from build123d import *

# Parameters (mm, degrees)
F1_DEPTH         = 50
F3_DEPTH         = 46
F5_DEPTH         = 25
F7_DEPTH         = 25
F8_W             = 3.4296980606
F8_H             = 1.9268138267
F9_DEPTH         = 25
F12_D            = 4
F12_DEPTH        = 16
F12_TIP          = 1.2017212381
F12_ON_F11_D     = 4
F12_ON_F11_DEPTH = 16
F12_ON_F11_TIP   = 1.2017212381
F13_R            = 5
F14_R            = 2
F15_R            = 5


with BuildPart() as f1:
    # F0 (on Right) → F1 (new body)
    with BuildSketch(Plane.YZ):
        Polygon((-50, 4), (-50, 0), (0, 0), (0, 50), (-4, 50), (-4, 4), align=None)
    extrude(amount=F1_DEPTH)

    # F2 (on face) → F3 (join)
    with BuildSketch(Plane.XZ.offset(4)):
        Polygon((25, 50), (24, 50), (24, 4), (26, 4), (26, 50), align=None)
    extrude(amount=F3_DEPTH)

    # F4 (on face) → F5 (cut)
    with BuildSketch(Plane(origin=(24, 0, 0), x_dir=(0, -1, 0), z_dir=(-1, 0, 0))):
        with BuildLine():
            Line((50, 50), (4, 50))
            add(Edge.make_bspline(
                [(4, 50), (18.2273147409, 34.0409380861), (26.0339638541, 8.7697255613), (37.7275896233, 4)],
                knots=[0, 0, 0, 0, 0.6888068808, 0.6888068808, 0.6888068808, 0.6888068808], degree=3))
            Line((37.7275896233, 4), (49.3700235132, 4))
            Line((49.3700235132, 4), (50, 4))
            Line((50, 4), (50, 50))
        make_face()
    extrude(amount=-F5_DEPTH, mode=Mode.SUBTRACT)

    # F6 (on face) → F7 (cut)
    with BuildSketch(Plane(origin=(24, 0, 0), x_dir=(0, -1, 0), z_dir=(-1, 0, 0))):
        with BuildLine():
            Line((4, 4), (20.8637948117, 4))
            add(Edge.make_bspline(
                [(20.8637948117, 4), (16.6060887277, 7.1307057515), (16.0147414533, 11.764077872), (13.590214774, 15.4687128961)],
                knots=[0, 0, 0, 0, 13.5807342238, 13.5807342238, 13.5807342238, 13.5807342238], degree=3))
            add(Edge.make_bspline(
                [(13.590214774, 15.4687128961), (8.6228903383, 18.1297790259), (5.6070159189, 17.9523732513), (4, 15.4687128961)],
                knots=[0, 0, 0, 0, 9.590214774, 9.590214774, 9.590214774, 9.590214774], degree=3))
            Line((4, 15.4687128961), (4, 4))
        make_face()
        Polygon((4, 33.209156245), (4, 24.3389345706), (10.5743389577, 24.3389345706), align=None)
    extrude(amount=-F7_DEPTH, mode=Mode.SUBTRACT)

    # F8 (on face) → F9 (cut)
    with BuildSketch(Plane(origin=(24, 0, 0), x_dir=(0, -1, 0), z_dir=(-1, 0, 0))):
        with Locations((5.7148490303, 16.4321198095)):
            Rectangle(F8_W, F8_H)
    extrude(amount=-F9_DEPTH, mode=Mode.SUBTRACT)

    # F12
    with Locations(Plane.XZ.offset(4)):
        with Locations((12.5, 27), (38, 27)):
            Hole(F12_D / 2, depth=F12_DEPTH)
            with Locations((0, 0, -(F12_DEPTH + F12_TIP / 2))):  # 118° drill point
                Cone(0, F12_D / 2, F12_TIP, mode=Mode.SUBTRACT)

    # F12 on F11
    with Locations(Plane.XY.offset(4)):
        with Locations((38, -27), (12, -27)):
            Hole(F12_ON_F11_D / 2, depth=F12_ON_F11_DEPTH)
            with Locations((0, 0, -(F12_ON_F11_DEPTH + F12_ON_F11_TIP / 2))):  # 118° drill point
                Cone(0, F12_ON_F11_D / 2, F12_ON_F11_TIP, mode=Mode.SUBTRACT)

    # F13
    f13_edges = [f1.edges().sort_by_distance(p)[0] for p in [
        (25, 0, 0),
    ]]
    fillet(f13_edges, radius=F13_R)

    # F14
    f14_edges = [f1.edges().sort_by_distance(p)[0] for p in [
        (25, -4, 4),
    ]]
    fillet(f14_edges, radius=F14_R)

    # F15
    f15_edges = [f1.edges().sort_by_distance(p)[0] for p in [
        (0, -2, 50),
        (50, -2, 50),
        (0, -50, 2),
        (50, -50, 2),
    ]]
    fillet(f15_edges, radius=F15_R)


solid = f1.part
Geometry check sheet. Reference: the model listing, model coordinates, mm. A direction names the side the tool comes from. Coordinates: 2 decimals unless noted, no trailing zeros. Order: outer loops, then holes, each group sorted by start corner. A loop starts at its lowest first (then second) coordinate and runs counter-clockwise, first axis right, second up. Notation, with made-up numbers: (-18, 43) - (27, 43) arc R11 cw to (27, 56) - close; hole circle Ø4 at (11.5, 63). An arc over 180 degrees is marked (long way). Answer in a Markdown table with one row per item. Add a question column.
1) Cross-section at C-C, the plane y = -27. State how many separate pieces and enclosed holes the cut face has, then the cut area to 3 significant figures.
2) Material ranges on line 1 along Y through (x, z) = (10.5, 38.5); line 2 along Z through (x, y) = (15, -7.5); line 3 along Z through (x, y) = (12, -1), recorded low to high. Write a range as [from, to].
3) Set-up check for faces 4 (the flat face through (25, -6, 17.396)), 5 (the cylindrical face through (1, -48, 2)), 6 (the flat face through (24, -16, 24)): record each of +Z, -Z, +X, -X, +Y, -Y from which the full face is reachable in a straight line by a thin tool's end or side.
4) Cross-section at B-B, the plane x = 15.5. Record the cut outline in (y, z), then the cut area to 3 significant figures.
5) Cross-section at A-A, the plane x = 38. Record the cut outline in (y, z).
6) Gauge pin test, flat ends, axial feed: P1, Ø4.5, axis at x = 38, y = -27, coming from the -Z side; P2, Ø4, axis at x = 7.5, y = -33.5, coming from the +Z side; P3, Ø1, axis at x = 30, z = 20, coming from the -Y side; P4, Ø17, axis at y = -17, z = 37, coming from the -X side. Record the tip position at first contact, or that the pin passes through.
7) Release check for a two-part mould opening along X. For faces 1 (the cylindrical face through (38, -2, 25)), 2 (the flat face through (25, -28, 0)), 3 (the cylindrical face through (48, -2, 49)) record: +X half, -X half, draft (parallel to the pull), parting line (faces both ways), or undercut.
8) Cross-section at D-D, the plane y = -39.5. Record the cut outline in (x, z), then the cut area to 3 significant figures.
Check result:
| question | item | result |
|---|---|---|
| 1 | separate pieces | 3 |
| 1 | enclosed holes | 0 |
| 1 | area | 189 mm² |
| 2 | line 1 | y = [-4, 0] |
| 2 | line 2 | z = [0, 4] |
| 2 | line 3 | z = [2, 25.06], [28.94, 50] |
| 3 | face 4 | +X, -X |
| 3 | face 5 | +Z, -Z, -X, -Y |
| 3 | face 6 | +Z, -X, -Y |
| 4 | outline | (-50, 0) - (-5, 0) arc R5 ccw to (0, 5) - (0, 50) - (-4, 50) - (-4, 6) arc R2 cw to (-6, 4) - (-50, 4) - close |
| 4 | area | 379 mm² |
| 5 | outline | (-50, 0) - (-29, 0) - (-29, 4) - (-50, 4) - close; (-25, 0) - (-5, 0) arc R5 ccw to (0, 5) - (0, 25) - (-4, 25) - (-4, 6) arc R2 cw to (-6, 4) - (-25, 4) - close; (-4, 29) - (0, 29) - (0, 50) - (-4, 50) - close |
| 6 | P1 | stops at z = 0 |
| 6 | P2 | stops at z = 4 |
| 6 | P3 | stops at y = -4 |
| 6 | P4 | stops at x = 24 |
| 7 | face 1 | undercut |
| 7 | face 2 | draft |
| 7 | face 3 | +X half |
| 8 | outline | (0, 0) - (50, 0) - (50, 4) - (0, 4) - close |
| 8 | area | 200 mm² |
